Verification items for the finished model (mm, model axes). A direction names the side the tool comes from. Give positions to 0.01 mm unless a question says otherwise; leave off trailing zeros. Order: outer loops, then holes, each group sorted by start corner. A loop starts at its lowest first (then second) coordinate and runs counter-clockwise, first axis right, second up. Notation, with made-up numbers: (48.5, -3) -> (92.5, -3) arc R32 cw to (92.5, 27) -> close; hole circle Ø9 at (0.5, 65.25). An arc over 180 degrees is marked (long way). Return JSON: item names as keys, results as strings. Group by question number.
(1) Cross-section at C-C on x = 3.81. Enter the section's corners in (y, z), then the cut area to 3 significant figures.
(2) Cross-section at B-B on y = -4.5. Enter the section's corners in (x, z).
(3) Cross-section at D-D on y = -3. Enter the section's corners in (x, z).
(4) Thickness scan on line 1 along Z through (x, y) = (-1, 2.5); line 2 along Y through (x, z) = (-1.25, -0.5); line 3 along Z through (x, y) = (-10, -4.25). Record the ranges inside material, lowest first.
(5) Tool access check on faces 4 (the face through (11, 0, 7.5)), 5 (the face through (0, 0, 8)). Record the directions out of +Z, -Z, +X, -X, +Y, -Y that give a thin tool (end or side, any length) a straight path to the whole face; none if there is none.
(6) Depth check by flat-ended pin: pin 1 Ø4 at (x, y) = (-1.5, -1) entering from -Z; pin 2 Ø0.5 at (x, y) = (-9, -1) entering from +Z. Enter the tip coordinate at first touch or a pass-through.
(7) Cross-section at A-A on x = -5.75. Enter the section's corners in (y, z), then the cut area to 3 significant figures.
(8) Release check for a two-part mould opening along X. For faces 1 (the face through (12.7, 0, 4)), 2 (the face through (-4, 0, 7.5)), 3 (the face through (0, 5.08, 4)) record: pulls with the +X half, pulls with the -X half, needs draft (parallel to the pull), parting line crosses it, or undercut.
from build123d import *

# Parameters (mm, degrees)
SALIENTE_EXTRUIR1_DEPTH = 8
CROQUIS3_R              = 0.25
SALIENTE_EXTRUIR2_DEPTH = 3
MATRIZL1_COUNT          = 2
MATRIZL1_PITCH          = 12.7
MATRIZL1_COUNT_DIR2     = 2
MATRIZL1_PITCH_DIR2     = 7.5
CROQUIS4_W              = 1.74
CROQUIS4_H              = 5.08
CORTAR_EXTRUIR1_DEPTH   = 0.5
MATRIZL2_COUNT          = 10
MATRIZL2_PITCH          = 2.54


with BuildPart() as part:
    # Croquis1 → Saliente-Extruir1 (new body)
    with BuildSketch(Plane.XY):
        Polygon((-11.7, -5.08), (-12.7, -4.08), (-12.7, 5.08), (12.7, 5.08), (12.7, -5.08), align=None)
    extrude(amount=SALIENTE_EXTRUIR1_DEPTH)

    # Croquis3 → Saliente-Extruir2 (add)
    with BuildSketch(Plane(origin=(0, 0, 0), x_dir=(-1, 0, 0), z_dir=(0, 0, -1))):
        with Locations((-11.43, 3.75)):
            Circle(CROQUIS3_R)
        with Locations((-8.89, 3.75)):
            Circle(CROQUIS3_R)
        with Locations((-6.35, 3.75)):
            Circle(CROQUIS3_R)
        with Locations((-3.81, 3.75)):
            Circle(CROQUIS3_R)
        with Locations((-1.27, 3.75)):
            Circle(CROQUIS3_R)
    saliente_extruir2 = extrude(amount=SALIENTE_EXTRUIR2_DEPTH)

    # MatrizL1: Saliente-Extruir2 2 × 2
    with Locations(*[(-i * MATRIZL1_PITCH, -j * MATRIZL1_PITCH_DIR2, 0) for i in range(MATRIZL1_COUNT) for j in range(MATRIZL1_COUNT_DIR2) if (i, j) != (0, 0)]):
        add(saliente_extruir2)

    # Croquis4 → Cortar-Extruir1 (cut)
    with BuildSketch(Plane.XY.offset(8)):
        with Locations((11.43, 0)):
            Rectangle(CROQUIS4_W, CROQUIS4_H)
    cortar_extruir1 = extrude(amount=-CORTAR_EXTRUIR1_DEPTH, mode=Mode.SUBTRACT)

    # MatrizL2: Cortar-Extruir1 ×10
    with Locations(*[(-i * MATRIZL2_PITCH, 0, 0) for i in range(1, MATRIZL2_COUNT)]):
        add(cortar_extruir1, mode=Mode.SUBTRACT)


solid = part.part
Verdict:
{
 "1": {"outline": "(-5.08, 0) -> (-4, 0) -> (-4, -3) -> (-3.5, -3) -> (-3.5, 0) -> (3.5, 0) -> (3.5, -3) -> (4, -3) -> (4, 0) -> (5.08, 0) -> (5.08, 8) -> (2.54, 8) -> (2.54, 7.5) -> (-2.54, 7.5) -> (-2.54, 8) -> (-5.08, 8) -> close", "area": "81.7 mm²"},
 "2": {"outline": "(-12.28, 0) -> (12.7, 0) -> (12.7, 8) -> (-12.28, 8) -> close"},
 "3": {"outline": "(-12.7, 0) -> (12.7, 0) -> (12.7, 8) -> (-12.7, 8) -> close"},
 "4": {"line 1": "0 to 7.5", "line 2": "-4 to -3.5, 3.5 to 4", "line 3": "0 to 8"},
 "5": {"face 4": "+Z", "face 5": "+Z, +X, -X, +Y, -Y"},
 "6": {"pin 1": "z = 0", "pin 2": "z = 7.5"},
 "7": {"outline": "(-5.08, 0) -> (5.08, 0) -> (5.08, 8) -> (2.54, 8) -> (2.54, 7.5) -> (-2.54, 7.5) -> (-2.54, 8) -> (-5.08, 8) -> close", "area": "78.7 mm²"},
 "8": {"face 1": "pulls with the +X half", "face 2": "undercut", "face 3": "needs draft"}
}
